The model under review builds one solid part; all positions refer to its coordinate system, in mm. Round coordinates to 2 decimals unless told otherwise and drop trailing zeros. Order: outer loops, then holes, each group sorted by start corner. A loop starts at its lowest first (then second) coordinate and runs counter-clockwise, first axis right, second up. Notation, with made-up numbers: M -38,69 L -6,69 A12 cw -6,92 Z; hole C 22,31.5 d3. An arc over 180 degrees is marked long. Answer as a JSON object with one key per item and string values. Group by question number.
1. Clearance check with flat-ended pins moving along their axes: P1, Ø5, axis at x = -108.63, z = -254.74, coming from the -Y side; P2, Ø2.5, axis at x = 313, y = -110, coming from the +Z side. State where each tip first meets the part, or that it passes through.
2. To check wall thickness, follow probe 1 along Z at (x, y) = (165.5, -112.1); probe 2 along Z at (x, y) = (-106, -110.35); probe 3 along Z at (x, y) = (-230.5, -112.2). State the ranges of each line that lie inside material, in increasing order. Write a range as [from, to].
3. Add section A-A on y = -110.4. Give the number of separate pieces and of enclosed holes in the cut face, and give its area (3 significant figures).
4. Add section B-B on z = -210.5. State the section outline as (x, y) points, and give its area (3 significant figures).
5. Add section C-C on x = 253.5. State the section outline as (y, z) points, and give its area (3 significant figures).
```python
from build123d import *

# Parameters (mm, degrees)
SKETCH2_R           = 4
BOSS_EXTRUDE1_DEPTH = 5
FILLET1_R           = 40


with BuildPart() as part:
    # Sketch2 → Boss-Extrude1 (new body)
    with BuildSketch(Plane(origin=(0, -112.700994014, 0), x_dir=(1, 0, 0), z_dir=(0, 1, 0))):
        Polygon((-188.563755175, 274.737493623), (244.595772671, 274.737493623), (244.595772671, 194.737493623), (324.595772671, 194.737493623), (324.595772671, -265.262506377), (244.595772671, -265.262506377), (244.595772671, -345.262506377), (-188.563755175, -345.262506377), (-188.563755175, -265.262506377), (-268.563755175, -265.262506377), (-268.563755175, 194.737493623), (-188.563755175, 194.737493623), align=None)
        with Locations(Location((-169.208419226, 254.737493623, 0), (0, 0, 270))):
            Circle(SKETCH2_R, mode=Mode.SUBTRACT)
        with Locations(Location((-108.626011264, 254.737493623, 0), (0, 0, 270))):
            Circle(SKETCH2_R, mode=Mode.SUBTRACT)
        with Locations(Location((-248.563755175, 188.837673249, 0), (0, 0, 270))):
            Circle(SKETCH2_R, mode=Mode.SUBTRACT)
        with Locations(Location((-248.563755175, 109.252031995, 0), (0, 0, 270))):
            Circle(SKETCH2_R, mode=Mode.SUBTRACT)
        with Locations(Location((304.595772671, 109.252031995, 0), (0, 0, 90))):
            Circle(SKETCH2_R, mode=Mode.SUBTRACT)
        with Locations(Location((164.658028761, 254.737493623, 0), (0, 0, 90))):
            Circle(SKETCH2_R, mode=Mode.SUBTRACT)
        with Locations(Location((225.240436722, 254.737493623, 0), (0, 0, 90))):
            Circle(SKETCH2_R, mode=Mode.SUBTRACT)
        with Locations(Location((304.595772671, 188.837673249, 0), (0, 0, 90))):
            Circle(SKETCH2_R, mode=Mode.SUBTRACT)
        with Locations(Location((304.595772671, -259.362686002, 0), (0, 0, 270))):
            Circle(SKETCH2_R, mode=Mode.SUBTRACT)
        with Locations(Location((225.240436722, -325.262506377, 0), (0, 0, 270))):
            Circle(SKETCH2_R, mode=Mode.SUBTRACT)
        with Locations(Location((164.658028761, -325.262506377, 0), (0, 0, 270))):
            Circle(SKETCH2_R, mode=Mode.SUBTRACT)
        with Locations(Location((304.595772671, -179.777044749, 0), (0, 0, 270))):
            Circle(SKETCH2_R, mode=Mode.SUBTRACT)
        with Locations(Location((-248.563755175, -179.777044749, 0), (0, 0, 90))):
            Circle(SKETCH2_R, mode=Mode.SUBTRACT)
        with Locations(Location((-248.563755175, -259.362686002, 0), (0, 0, 90))):
            Circle(SKETCH2_R, mode=Mode.SUBTRACT)
        with Locations(Location((-108.626011264, -325.262506377, 0), (0, 0, 90))):
            Circle(SKETCH2_R, mode=Mode.SUBTRACT)
        with Locations(Location((-169.208419226, -325.262506377, 0), (0, 0, 90))):
            Circle(SKETCH2_R, mode=Mode.SUBTRACT)
    extrude(amount=BOSS_EXTRUDE1_DEPTH)

    # Fillet1
    fillet1_edges = [part.edges().sort_by_distance(p)[0] for p in [
        (244.595772671, -110.200994014, -194.737493623),
        (244.595772671, -110.200994014, 265.262506377),
        (-188.563755175, -110.200994014, 265.262506377),
        (-188.563755175, -110.200994014, -194.737493623),
    ]]
    fillet(fillet1_edges, radius=FILLET1_R)


solid = part.part
```
Recorded:
{
 "1": {"P1": "passes through", "P2": "stops at z = 265.26"},
 "2": {"probe 1": "z = [-274.74, -258.65], [-250.83, 321.35], [329.17, 345.26]", "probe 2": "z = [-274.74, -257.75], [-251.72, 322.25], [328.28, 345.26]", "probe 3": "z = [-194.74, 265.26]"},
 "3": {"separate pieces": "1", "enclosed holes": "16", "area": "343,000 mm²"},
 "4": {"outline": "M -196.74,-112.7 L 252.78,-112.7 L 252.78,-107.7 L -196.74,-107.7 Z", "area": "2,250 mm²"},
 "5": {"outline": "M -112.7,-209.58 L -107.7,-209.58 L -107.7,280.1 L -112.7,280.1 Z", "area": "2,450 mm²"}
}
